Can you work these out from the model? Positions are in its coordinate system, mm. Face numbers are marked on the shaded views. A direction names the side the tool comes from. Coordinates: 2 decimals unless noted, no trailing zeros. Order: outer loops, then holes, each group sorted by start corner. A loop starts at its lowest first (then second) coordinate and runs counter-clockwise, first axis right, second up. Notation, with made-up numbers: (79, 37) -> (137, 37) arc R20 ccw to (137, 46) -> close; hole circle Ø6 at (-34, -37.75). An arc over 180 degrees is marked (long way). Return JSON: item names as keys, results as strings. Group by question number.
1) If I drill on probe 1 along Y at (x, z) = (0, -17); probe 2 along Z at (x, y) = (3.75, 1); probe 3 along Y at (x, z) = (2, -24.5), over which ranges is the centre line in solid material (lowest first)? Write a range as from..to.
2) For the marked faces 1, 2 and 3, which set-ups out of +Z, -Z, +X, -X, +Y, -Y let a thin tool reach every point of the face, with its end or its side?
3) If we section it at C-C, the plane z = -10.5: Please give me the cut outline in (x, y).
4) If we section it at D-D, the plane z = -24.75: Please give me the cut outline in (x, y).
5) For pin 1 (4 mm diameter, centred on y = 4, z = -23, fed in from +X); pin 2 (4 mm diameter, centred on x = 3.5, z = -19.5, fed in from +Y); pin 3 (6 mm diameter, centred on y = -2, z = -7, fed in from -X), each with a flat end and sliding along its axis, tell me the tip position at first contact or that it passes through.
6) If we section it at A-A, the plane x = 0: Please give me the cut outline in (y, z).
7) If we section it at B-B, the plane y = 0: Please give me the cut outline in (x, z), then the cut area to 3 significant figures.
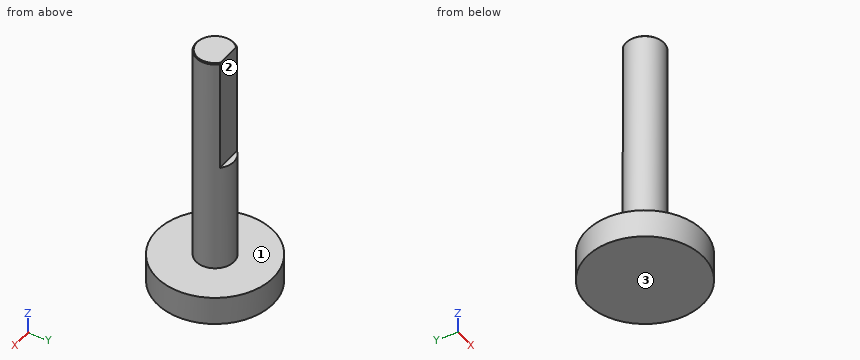
from build123d import *

# Parameters (mm, degrees)
SKETCH1_R           = 2
BOSS_EXTRUDE1_DEPTH = 26.5
SKETCH2_R           = 6.15
BOSS_EXTRUDE2_DEPTH = 3
CHAMFER1_SIZE       = 0.1
CUT_EXTRUDE2_DEPTH  = 12


with BuildPart() as part:
    # Sketch1 → Boss-Extrude1 (new body)
    with BuildSketch(Plane.XY):
        Circle(SKETCH1_R)
    extrude(amount=-BOSS_EXTRUDE1_DEPTH)

    # Sketch2 → Boss-Extrude2 (add)
    with BuildSketch(Plane(origin=(0, 0, -26.5), x_dir=(-1, 0, 0), z_dir=(0, 0, -1))):
        Circle(SKETCH2_R)
    extrude(amount=-BOSS_EXTRUDE2_DEPTH)

    # Chamfer1
    chamfer1_edges = [part.edges().sort_by_distance(p)[0] for p in [
        (-2, 0, 0),
    ]]
    chamfer(chamfer1_edges, length=CHAMFER1_SIZE)

    # Sketch3 → Cut-Extrude2 (cut)
    with BuildSketch(Plane.XY):
        with BuildLine():
            Line((1.428285686, 1.4), (-1.428285686, 1.4))
            ThreePointArc((-1.428285686, 1.4), (0, 2), (1.428285686, 1.4))
        make_face()
    extrude(amount=-CUT_EXTRUDE2_DEPTH, mode=Mode.SUBTRACT)


solid = part.part
Result sheet:
{
 "1": {"probe 1": "y = -2..2", "probe 2": "z = -26.5..-23.5", "probe 3": "y = -5.82..5.82"},
 "2": {"face 1": "+Z", "face 2": "+Z, +X, -X, +Y", "face 3": "-Z, +X, -X, +Y, -Y"},
 "3": {"outline": "(-1.43, 1.4) arc R2 ccw (long way) to (1.43, 1.4) -> close"},
 "4": {"outline": "circle Ø12.3 at (0, 0)"},
 "5": {"pin 1": "stops at x = 5.79", "pin 2": "stops at y = 1.32", "pin 3": "stops at x = -2"},
 "6": {"outline": "(-6.15, -26.5) -> (6.15, -26.5) -> (6.15, -23.5) -> (2, -23.5) -> (2, -12) -> (1.4, -12) -> (1.4, 0) -> (-1.9, 0) -> (-2, -0.1) -> (-2, -23.5) -> (-6.15, -23.5) -> close"},
 "7": {"outline": "(-6.15, -26.5) -> (6.15, -26.5) -> (6.15, -23.5) -> (2, -23.5) -> (2, -0.1) -> (1.9, 0) -> (-1.9, 0) -> (-2, -0.1) -> (-2, -23.5) -> (-6.15, -23.5) -> close", "area": "131 mm2"}
}
